Check sheet for the modelled part. Datum: model origin and axes. Units: mm. Coordinates: 2 decimals unless noted, no trailing zeros. Loops run counter-clockwise (first coordinate to the right, second up) from the corner with the lowest first, then second, coordinate; pieces in that order, holes last. Notation, with made-up numbers: (3, 57.5) -> (14, 57.5) arc R8 cw to (14, 65.5) -> close; hole circle Ø3 at (32, 79.5). An arc over 180 degrees is marked (long way). Use one line per item in the form item = value.
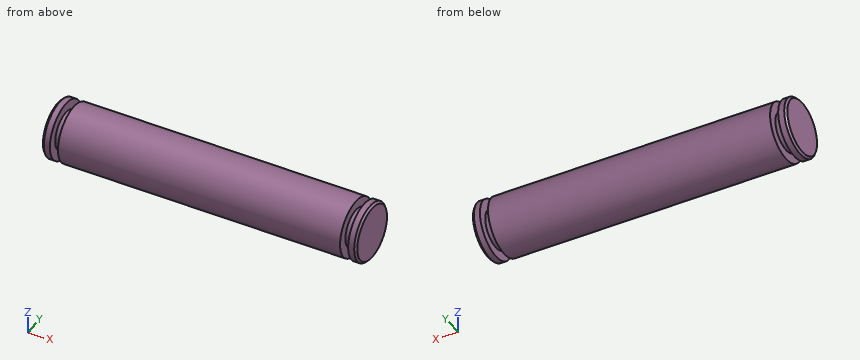
Autodesk Inventor part; units mm, degrees
ref_plane "YZ Plane" through (0, 0, 0) normal (1, 0, 0) x (0, 1, 0)
ref_plane "XZ Plane" through (0, 0, 0) normal (0, 1, 0) x (-1, 0, 0)
ref_plane "XY Plane" through (0, 0, 0) normal (0, 0, 1) x (1, 0, 0)
sketch "Esboço2" plane through (0, 0, 0) normal (1, 0, 0) x (0, 1, 0)
  circle A0 centre (0, 0) radius 7.1437
  dimension "d0" = 14.2875
extrude "Extrusão1" add sketch "Esboço2" along normal blind 2
sketch "Esboço3" plane through (2, 0, 0) normal (1, 0, 0) x (0, 0, -1)
  circle A0 centre (0, 0) radius 7.1437
  circle A1 centre (0, 0) radius 4.7625
  dimension "d3" = 9.525
extrude "Extrusão2" add sketch "Esboço3" along normal blind 2 contours A1
sketch "Esboço4" plane through (4, 0, 0) normal (1, 0, 0) x (0, 0, -1)
  circle A0 centre (0, 0) radius 4.7625
  circle A1 centre (0, 0) radius 7.1437
  dimension "d6" = 14.2875
extrude "Extrusão3" add sketch "Esboço4" along normal blind 70 contours A0 | A1
sketch "Esboço5" plane through (74, 0, 0) normal (1, 0, 0) x (0, 0, -1)
  circle A0 centre (0, 0) radius 7.1437
  circle A1 centre (0, 0) radius 4.7625
  dimension "d9" = 9.525
extrude "Extrusão4" add sketch "Esboço5" along normal blind 2 contours A1
sketch "Esboço6" plane through (76, 0, 0) normal (1, 0, 0) x (0, 0, -1)
  circle A0 centre (0, 0) radius 4.7625
  circle A1 centre (0, 0) radius 7.1437
  dimension "d12" = 14.2875
extrude "Extrusão5" add sketch "Esboço6" along normal blind 2 contours A0 | A1
chamfer "Chanfro1" distance 0.5 angle 45 2 edges at (0, -7.1437, 0) (78, 0, 7.1437)
properties part number "pino_a3" material "Aço carbono"
(1) Section check C-C, the plane x = 55.5. Record the boundary of the cut face in (y, z).
Established:
outline = circle Ø14.29 at (0, 0)
(2) Section check A-A, the plane z = 0. Record the boundary of the cut face in (x, y), plus the area to 3 significant figures.
Established:
outline = (0, -6.64) -> (0.5, -7.14) -> (2, -7.14) -> (2, -4.76) -> (4, -4.76) -> (4, -7.14) -> (74, -7.14) -> (74, -4.76) -> (76, -4.76) -> (76, -7.14) -> (77.5, -7.14) -> (78, -6.64) -> (78, 6.64) -> (77.5, 7.14) -> (76, 7.14) -> (76, 4.76) -> (74, 4.76) -> (74, 7.14) -> (4, 7.14) -> (4, 4.76) -> (2, 4.76) -> (2, 7.14) -> (0.5, 7.14) -> (0, 6.64) -> close
area = 1,090 mm²
(3) Scan lines: line 1 along X through (y, z) = (5, 3.25); line 2 along X through (y, z) = (-2.5, 6.25); line 3 along Y through (x, z) = (47, -0.25). Record each from-to range of solid material in increasing order.
Established:
line_1 = 0 to 2, 4 to 74, 76 to 78
line_2 = 0.09 to 2, 4 to 74, 76 to 77.91
line_3 = -7.14 to 7.14
(4) Go/stop test with flat-tipped pins: P1, Ø1.5, axis at x = 66.5, y = -2, coming from the +Z side; P2, Ø1.5, axis at x = 51, y = -5.5, coming from the -Z side; P3, Ø1.5, axis at x = 52.5, z = -4, coming from the +Y side. Record where each tip stops, or that it passes through.
Established:
P1 = 7.03
P2 = -5.34
P3 = 6.36
